CAD build for the part. Positions are in the model's coordinates, mm. A direction names the side the tool comes from. Give positions to 0.01 mm unless a question says otherwise; leave off trailing zeros. Order: outer loops, then holes, each group sorted by start corner. A loop starts at its lowest first (then second) coordinate and runs counter-clockwise, first axis right, second up. Notation, with made-up numbers: (31, 70) -> (59, 70) arc R20 ccw to (59, 87) -> close; hole circle Ø4 at (11.25, -6.5). An arc over 180 degrees is marked (long way). Use one line per item in the form item = value. Start each with the question number.
1) Cut at B-B, the plane x = 262. Give the cut face in (y, z) (3 decimals).
2) Tool access for faces 3 (the face through (-10, 10, 76.2)), 4 (the face through (-10, -10, 76.2)), 5 (the face through (219, 0, 79.375)), 6 (the face through (455, -10, 76.2)), 7 (the face through (16, -1, 0)): list every direction of +Z, -Z, +X, -X, +Y, -Y with a clear straight run to the whole face (end or side of a thin tool).
3) Cut at C-C, the plane x = 198. Give the cut face in (y, z) (3 decimals), and give its area (3 significant figures).
4) Mould opens along X. For faces 1 (the face through (175, -1, 0)), 2 (the face through (454, 10, 76.2)) say: pulls with the +X half, pulls with the -X half, needs draft (parallel to the pull), parting line crosses it, or undercut.
5) Probe line 1 (Y direction, x = 31.75, z = 62) (3 decimals); line 2 (Z direction, x = 393.5, y = -7.5) (3 decimals); line 3 (Y direction, x = 103, z = 57). List the from-to ranges inside material, lowest first.
6) Cut at A-A, the plane z = 28.5. State how many separate pieces and enclosed holes the cut face has, and give its area (3 significant figures).
7) Drop flat-ended pins along their axis: P1, Ø4, axis at x = 324.5, z = 70, coming from the -Y side; P2, Ø8, axis at y = -7.5, z = 22, coming from the -X side; P3, Ø4, axis at x = 42, z = 23.5, coming from the -Y side; P4, Ø4, axis at x = 111, z = 46, coming from the +Y side. Give the stop position or say it passes through.
from build123d import *

# Parameters (mm, degrees)
SKETCH1_R           = 12.7
BOSS_EXTRUDE1_DEPTH = 76.2
LPATTERN1_COUNT     = 15
LPATTERN1_PITCH     = 31.75
SKETCH2_W           = 469.9
SKETCH2_H           = 25.4
BOSS_EXTRUDE2_DEPTH = 3.175
SKETCH3_R           = 8.255
CUT_EXTRUDE1_DEPTH  = 465.766212735


with BuildPart() as part:
    # Sketch1 → Boss-Extrude1 (new body)
    with BuildSketch(Plane.XY):
        with Locations(Location((0, 0, 0), (0, 0, 180))):
            Circle(SKETCH1_R)
    extrude(amount=BOSS_EXTRUDE1_DEPTH)


with BuildPart() as lpattern1_1:
    # LPattern1: pattern copy
    add(part.part.moved(Location(Vector(1, 0, 0) * (1 * LPATTERN1_PITCH))))


with BuildPart() as lpattern1_2:
    # LPattern1: pattern copy
    add(part.part.moved(Location(Vector(1, 0, 0) * (2 * LPATTERN1_PITCH))))


with BuildPart() as lpattern1_3:
    # LPattern1: pattern copy
    add(part.part.moved(Location(Vector(1, 0, 0) * (3 * LPATTERN1_PITCH))))


with BuildPart() as lpattern1_4:
    # LPattern1: pattern copy
    add(part.part.moved(Location(Vector(1, 0, 0) * (4 * LPATTERN1_PITCH))))


with BuildPart() as lpattern1_5:
    # LPattern1: pattern copy
    add(part.part.moved(Location(Vector(1, 0, 0) * (5 * LPATTERN1_PITCH))))


with BuildPart() as lpattern1_6:
    # LPattern1: pattern copy
    add(part.part.moved(Location(Vector(1, 0, 0) * (6 * LPATTERN1_PITCH))))


with BuildPart() as lpattern1_7:
    # LPattern1: pattern copy
    add(part.part.moved(Location(Vector(1, 0, 0) * (7 * LPATTERN1_PITCH))))


with BuildPart() as lpattern1_8:
    # LPattern1: pattern copy
    add(part.part.moved(Location(Vector(1, 0, 0) * (8 * LPATTERN1_PITCH))))


with BuildPart() as lpattern1_9:
    # LPattern1: pattern copy
    add(part.part.moved(Location(Vector(1, 0, 0) * (9 * LPATTERN1_PITCH))))


with BuildPart() as lpattern1_10:
    # LPattern1: pattern copy
    add(part.part.moved(Location(Vector(1, 0, 0) * (10 * LPATTERN1_PITCH))))


with BuildPart() as lpattern1_11:
    # LPattern1: pattern copy
    add(part.part.moved(Location(Vector(1, 0, 0) * (11 * LPATTERN1_PITCH))))


with BuildPart() as lpattern1_12:
    # LPattern1: pattern copy
    add(part.part.moved(Location(Vector(1, 0, 0) * (12 * LPATTERN1_PITCH))))


with BuildPart() as lpattern1_13:
    # LPattern1: pattern copy
    add(part.part.moved(Location(Vector(1, 0, 0) * (13 * LPATTERN1_PITCH))))


with BuildPart() as lpattern1_14:
    # LPattern1: pattern copy
    add(part.part.moved(Location(Vector(1, 0, 0) * (14 * LPATTERN1_PITCH))))


with BuildPart() as part_1:
    add(part.part)

    add(lpattern1_1.part)  # Boss-Extrude2 merges LPattern1_1

    add(lpattern1_2.part)  # Boss-Extrude2 merges LPattern1_2

    add(lpattern1_3.part)  # Boss-Extrude2 merges LPattern1_3

    add(lpattern1_4.part)  # Boss-Extrude2 merges LPattern1_4

    add(lpattern1_5.part)  # Boss-Extrude2 merges LPattern1_5

    add(lpattern1_6.part)  # Boss-Extrude2 merges LPattern1_6

    add(lpattern1_7.part)  # Boss-Extrude2 merges LPattern1_7

    add(lpattern1_8.part)  # Boss-Extrude2 merges LPattern1_8

    add(lpattern1_9.part)  # Boss-Extrude2 merges LPattern1_9

    add(lpattern1_10.part)  # Boss-Extrude2 merges LPattern1_10

    add(lpattern1_11.part)  # Boss-Extrude2 merges LPattern1_11

    add(lpattern1_12.part)  # Boss-Extrude2 merges LPattern1_12

    add(lpattern1_13.part)  # Boss-Extrude2 merges LPattern1_13

    add(lpattern1_14.part)  # Boss-Extrude2 merges LPattern1_14
    # Sketch2 → Boss-Extrude2 (add)
    with BuildSketch(Plane.XY.offset(76.2)):
        with Locations((222.25, 0)):
            Rectangle(SKETCH2_W, SKETCH2_H)
    boss_extrude2 = extrude(amount=BOSS_EXTRUDE2_DEPTH)

    # Mirror1: Boss-Extrude2 across plane
    add(boss_extrude2.mirror(Plane.XY.offset(38.1)))

    # Sketch3 → Cut-Extrude1 (cut, through all)
    with BuildSketch(Plane.XY.offset(79.375)):
        with Locations((31.75, 0)):
            Circle(SKETCH3_R)
        Polygon((7.332348419, 0), (3.666174209, 6.35), (-3.666174209, 6.35), (-7.332348419, 0), (-3.666174209, -6.35), (3.666174209, -6.35), align=None)
    extrude(amount=-CUT_EXTRUDE1_DEPTH, mode=Mode.SUBTRACT)


solid = part_1.part
Result:
q1.outline = (-12.7, -3.175) -> (12.7, -3.175) -> (12.7, 0) -> (9.864, 0) -> (9.864, 76.2) -> (12.7, 76.2) -> (12.7, 79.375) -> (-12.7, 79.375) -> (-12.7, 76.2) -> (-9.864, 76.2) -> (-9.864, 0) -> (-12.7, 0) -> close
q2.face_3 = -X, +Y
q2.face_4 = -X, -Y
q2.face_5 = +Z, +X, -X, +Y, -Y
q2.face_6 = +X, -Y
q2.face_7 = none
q3.outline = (-12.7, -3.175) -> (12.7, -3.175) -> (12.7, 0) -> (10.249, 0) -> (10.249, 76.2) -> (12.7, 76.2) -> (12.7, 79.375) -> (-12.7, 79.375) -> (-12.7, 76.2) -> (-10.249, 76.2) -> (-10.249, 0) -> (-12.7, 0) -> close
q3.area = 1,720 mm²
q4.face_1 = undercut
q4.face_2 = needs draft
q5.line_1 = -12.7 to -8.255, 8.255 to 12.7
q5.line_2 = -3.175 to 0, 76.2 to 79.375
q5.line_3 = -10.06 to 10.06
q6.separate_pieces = 15
q6.enclosed_holes = 2
q6.area = 7,250 mm²
q7.P1 = -11.67
q7.P2 = -12.21
q7.P3 = -9.66
q7.P4 = through
